Input: part model. Units: mm. Frame: model coordinates. Face numbers are marked on the shaded views. A direction names the side the tool comes from. Give positions to 0.01 mm unless a question says otherwise; leave off trailing zeros. Order: outer loops, then holes, each group sorted by start corner. A loop starts at its lowest first (then second) coordinate and runs counter-clockwise, first axis right, second up. Notation, with made-up numbers: (53, 55) - (86, 55) arc R29 cw to (86, 75) - close; hole circle Ø3 at (-28.5, -33.5). An arc over 180 degrees is marked (long way). Use a Markdown table: item, result.
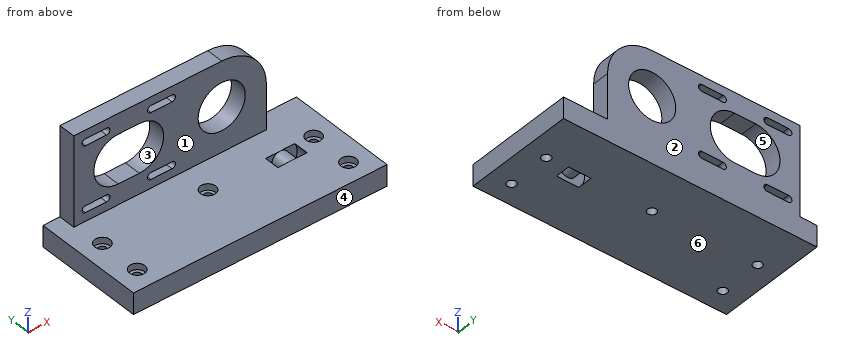
from build123d import *

# Parameters (mm, degrees)
CYLINDER001_R     = 4
CYLINDER001_DEPTH = 10
CYLINDER_R        = 8
CYLINDER_DEPTH    = 7
CUT_ROLL_ANGLE    = 90
SKETCH_W          = 120
SKETCH_H          = 52
SKETCH_R          = 2.1
PAD_DEPTH         = 10
SKETCH007_R       = 11.15
PAD001_DEPTH      = 8
SKETCH008_R       = 3.6
SKETCH008_R_2     = 2.1
POCKET_DEPTH      = 3


with BuildPart() as zylinder001:
    # Cylinder001 → Cylinder001 (new body)
    with BuildSketch(Plane.XY):
        Circle(CYLINDER001_R)
    extrude(amount=CYLINDER001_DEPTH)


with BuildPart() as cut:
    # Cylinder → Cylinder (new body)
    with BuildSketch(Plane.XY):
        Circle(CYLINDER_R)
    extrude(amount=CYLINDER_DEPTH)

    # Cut: cut Zylinder001
    add(zylinder001.part, mode=Mode.SUBTRACT)


with BuildPart() as cut_1:
    # Cut roll: moved
    add(cut.part.rotate(Axis((0, 0, 0), (1, 0, 0)), CUT_ROLL_ANGLE))


with BuildPart() as cut_2:
    # Cut placement: moved
    add(cut_1.part.moved(Location((35, 5, 6))))


with BuildPart() as cut001:
    # Sketch → Pad (new body)
    with BuildSketch(Plane.XY):
        Rectangle(SKETCH_W, SKETCH_H)
        with Locations((-50, -16)):
            Circle(SKETCH_R, mode=Mode.SUBTRACT)
        with Locations((-50, 4)):
            Circle(SKETCH_R, mode=Mode.SUBTRACT)
        with Locations((0, 4)):
            Circle(SKETCH_R, mode=Mode.SUBTRACT)
        with Locations((50, 4)):
            Circle(SKETCH_R, mode=Mode.SUBTRACT)
        with Locations((50, -16)):
            Circle(SKETCH_R, mode=Mode.SUBTRACT)
    extrude(amount=PAD_DEPTH)

    # Sketch007 → Pad001 (new body)
    with BuildSketch(Plane(origin=(0, 26, 0), x_dir=(-1, 0, 0), z_dir=(0, 1, 0))):
        with BuildLine():
            Line((0, 10), (52, 10))
            Line((52, 10), (52, 52.3))
            Line((52, 52.3), (0, 52.3))
            Line((0, 52.3), (-18.00006, 52.3))
            ThreePointArc((-18.00006, 52.3), (-32.95533, 46.105287), (-39.15, 31.15))
            Line((-39.15, 10), (-39.15, 31.15))
            Line((0, 10), (-39.15, 10))
        make_face()
        with Locations((-18, 31.15)):
            Circle(SKETCH007_R, mode=Mode.SUBTRACT)
        with BuildLine():
            ThreePointArc((21, 42.65), (9.5, 31.15), (21, 19.65))
            Line((21, 19.65), (31, 19.65))
            ThreePointArc((31, 19.65), (42.5, 31.15), (31, 42.65))
            Line((21, 42.65), (31, 42.65))
        make_face(mode=Mode.SUBTRACT)
        with BuildLine():
            ThreePointArc((36.5, 48.25), (34.9, 46.65), (36.5, 45.05))
            Line((36.5, 45.05), (46.5, 45.05))
            ThreePointArc((46.5, 45.05), (48.1, 46.65), (46.5, 48.25))
            Line((36.5, 48.25), (46.5, 48.25))
        make_face(mode=Mode.SUBTRACT)
        with BuildLine():
            ThreePointArc((5.5, 48.25), (3.9, 46.65), (5.5, 45.05))
            Line((5.5, 45.05), (15.5, 45.05))
            ThreePointArc((15.5, 45.05), (17.1, 46.65), (15.5, 48.25))
            Line((5.5, 48.25), (15.5, 48.25))
        make_face(mode=Mode.SUBTRACT)
        with BuildLine():
            ThreePointArc((5.5, 17.25), (3.9, 15.65), (5.5, 14.05))
            Line((5.5, 14.05), (15.5, 14.05))
            ThreePointArc((15.5, 14.05), (17.1, 15.65), (15.5, 17.25))
            Line((5.5, 17.25), (15.5, 17.25))
        make_face(mode=Mode.SUBTRACT)
        with BuildLine():
            ThreePointArc((36.5, 17.25), (34.9, 15.65), (36.5, 14.05))
            Line((36.5, 14.05), (46.5, 14.05))
            ThreePointArc((46.5, 14.05), (48.1, 15.65), (46.5, 17.25))
            Line((36.5, 17.25), (46.5, 17.25))
        make_face(mode=Mode.SUBTRACT)
    extrude(amount=-PAD001_DEPTH)

    # Sketch008 → Pocket (cut)
    with BuildSketch(Plane.XY.offset(10)):
        with Locations((-50, 4)):
            Circle(SKETCH008_R)
        with Locations((-50, 4)):
            Circle(SKETCH008_R_2, mode=Mode.SUBTRACT)
        with Locations((-50, -16)):
            Circle(SKETCH008_R)
        with Locations((-50, -16)):
            Circle(SKETCH008_R_2, mode=Mode.SUBTRACT)
        with Locations((0, 4)):
            Circle(SKETCH008_R)
        with Locations((0, 4)):
            Circle(SKETCH008_R_2, mode=Mode.SUBTRACT)
        with Locations((50, 4)):
            Circle(SKETCH008_R)
        with Locations((50, 4)):
            Circle(SKETCH008_R_2, mode=Mode.SUBTRACT)
        with Locations((50, -16)):
            Circle(SKETCH008_R)
        with Locations((50, -16)):
            Circle(SKETCH008_R_2, mode=Mode.SUBTRACT)
    extrude(amount=-POCKET_DEPTH, mode=Mode.SUBTRACT)

    # Cut001: cut Cut
    add(cut_2.part, mode=Mode.SUBTRACT)


solid = cut001.part
1. Material intervals for line 1 along Y through (x, z) = (50, 9); line 2 along Y through (x, z) = (-50, 4.5); line 3 along X through (y, z) = (21, 31), sorted ascending.
Response:
| item | result |
|---|---|
| line 1 | y = -26 to -19.6, -12.4 to 0.4, 7.6 to 26 |
| line 2 | y = -26 to -18.1, -13.9 to 1.9, 6.1 to 26 |
| line 3 | x = -52 to -42.5, -9.5 to 6.85, 29.15 to 39.15 |
2. Pin query (flat end, axial travel): pin 1 (3.5 mm diameter, centred on x = 50, y = 4, fed in from +Z); pin 2 (4 mm diameter, centred on y = 21.5, z = 25, fed in from +X); pin 3 (6 mm diameter, centred on x = 15.5, y = -18, fed in from +Z); pin 4 (9 mm diameter, centred on y = 20, z = 34, fed in from -X). Return the tip coordinate at first contact, or that it passes through.
Response:
| item | result |
|---|---|
| pin 1 | passes through |
| pin 2 | stops at x = 39.15 |
| pin 3 | stops at z = 10 |
| pin 4 | stops at x = -52 |
3. Section query D-D (z = 37.5). Return loops of the section in (x, y).
Response:
| item | result |
|---|---|
| outline | (-52, 18) - (-40.59, 18) - (-40.59, 26) - (-52, 26) - close; (-11.41, 18) - (8.83, 18) - (8.83, 26) - (-11.41, 26) - close; (27.17, 18) - (38.17, 18) - (38.17, 26) - (27.17, 26) - close |
4. Section query A-A (x = -28.5). Return loops of the section in (y, z), then the cut area to 3 significant figures.
Response:
| item | result |
|---|---|
| outline | (-26, 0) - (26, 0) - (26, 19.65) - (18, 19.65) - (18, 10) - (-26, 10) - close; (18, 42.65) - (26, 42.65) - (26, 52.3) - (18, 52.3) - close |
| area | 674 mm^2 |
5. Section query B-B (z = 29). Return loops of the section in (x, y), then the cut area to 3 significant figures.
Response:
| item | result |
|---|---|
| outline | (-52, 18) - (-42.3, 18) - (-42.3, 26) - (-52, 26) - close; (-9.7, 18) - (7.06, 18) - (7.06, 26) - (-9.7, 26) - close; (28.94, 18) - (39.15, 18) - (39.15, 26) - (28.94, 26) - close |
| area | 293 mm^2 |
6. Set-up query: the marked faces 1, 2 and 3. Return all of +Z, -Z, +X, -X, +Y, -Y with unobstructed straight access to the full face (end or side cutting, diameter ignored); none if empty.
Response:
| item | result |
|---|---|
| face 1 | +Z, +X, -X, -Y |
| face 2 | +Z, -Z, +X, -X, +Y |
| face 3 | +Y, -Y |
7. Mould query, pull axis Z, two halves, no side actions, for the marked faces 4, 5 and 6. Classes: pulls with the +Z half, pulls with the -Z half, needs draft (parallel to the pull), parting line crosses it, or undercut.
Response:
| item | result |
|---|---|
| face 4 | needs draft |
| face 5 | undercut |
| face 6 | pulls with the -Z half |
8. Section query C-C (x = -50). Return loops of the section in (y, z).
Response:
| item | result |
|---|---|
| outline | (-26, 0) - (-18.1, 0) - (-18.1, 7) - (-19.6, 7) - (-19.6, 10) - (-26, 10) - close; (-13.9, 0) - (1.9, 0) - (1.9, 7) - (0.4, 7) - (0.4, 10) - (-12.4, 10) - (-12.4, 7) - (-13.9, 7) - close; (6.1, 0) - (26, 0) - (26, 52.3) - (18, 52.3) - (18, 10) - (7.6, 10) - (7.6, 7) - (6.1, 7) - close |
